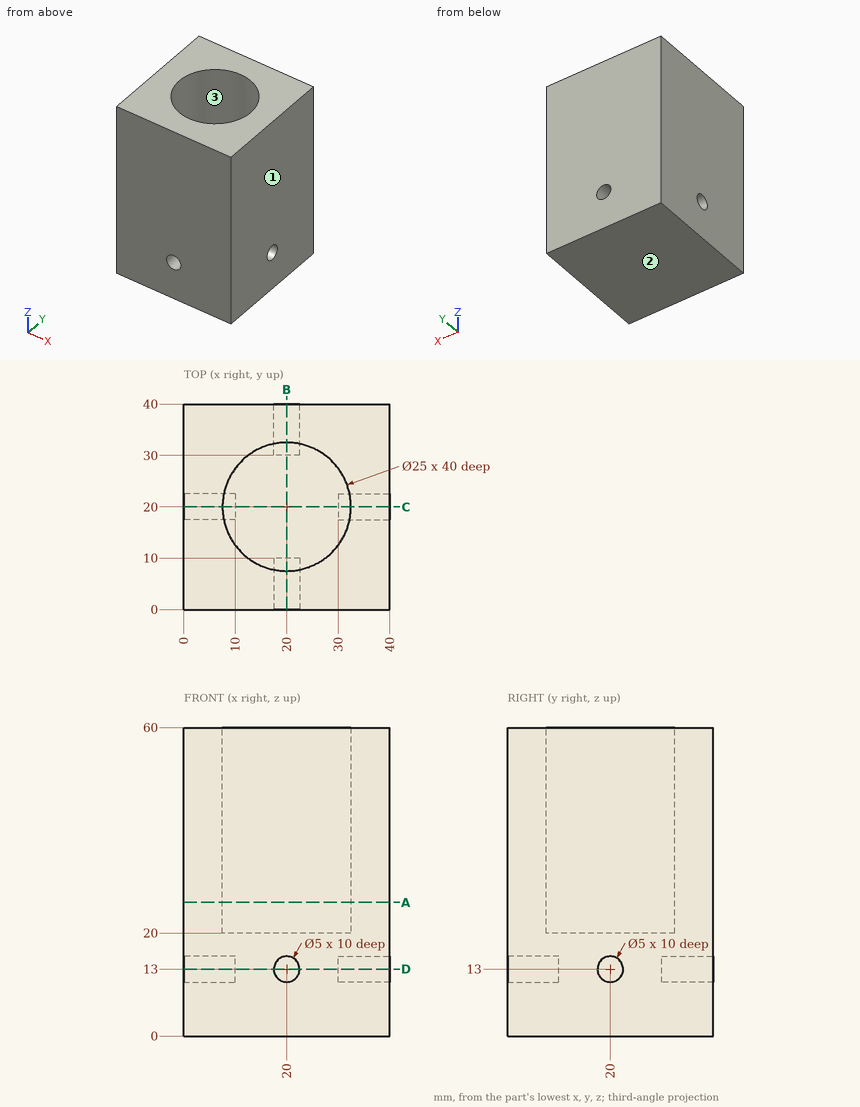
Answer from the drawing. Dimensions are ordinates in mm from the lowest x, y and z of the part. Give positions to 0.01 mm unless a question says otherwise; leave off trailing zeros. Order: outer loops, then holes, each group sorted by start corner. A loop starts at its lowest first (then second) coordinate and runs counter-clockwise, first axis right, second up. Notation, with made-up numbers: (-33, 63) -> (8, 63) arc R28 ccw to (8, 98) -> close; hole circle Ø10 at (21, 87.5). An arc over 180 degrees is marked (long way). One line per item, written item: value.
Item 1: Find section D-D, the plane z = 13. Give the vertices of the cut face in (x, y), plus the area to 3 significant figures.
Answer sheet:
outline: (0, 0) -> (17.5, 0) -> (17.5, 10) -> (22.5, 10) -> (22.5, 0) -> (40, 0) -> (40, 17.5) -> (30, 17.5) -> (30, 22.5) -> (40, 22.5) -> (40, 40) -> (22.5, 40) -> (22.5, 30) -> (17.5, 30) -> (17.5, 40) -> (0, 40) -> (0, 22.5) -> (10, 22.5) -> (10, 17.5) -> (0, 17.5) -> close
area: 1,400 mm²
Item 2: Find section A-A, the plane z = 26. Give the vertices of the cut face in (x, y).
Answer sheet:
outline: (0, 0) -> (40, 0) -> (40, 40) -> (0, 40) -> close; hole circle Ø25 at (20, 20)
Item 3: Flat-ended cylindrical pins translate along their axes: P1, Ø5, axis at x = 6, y = 8.5, coming from the -Z side; P2, Ø4, axis at y = 20, z = 13, coming from the +X side; P3, Ø12.5, axis at x = 19, y = 26, coming from the +Z side; P4, Ø1.5, axis at x = 19.5, z = 12, coming from the +Y side. Find the tip coordinate at first contact, or state that the pin passes through.
Answer sheet:
P1: z = 0
P2: x = 30
P3: z = 20
P4: y = 30
Item 4: Determine the mould class of the marked faces 1, 2 and 3 for opening direction X: released by +X, released by -X, zero draft, split by the parting line, or undercut.
Answer sheet:
face 1: released by +X
face 2: zero draft
face 3: undercut
Item 5: Straight lines are drawn through the part: probe 1 along Y at (x, z) = (12.5, 44.5); probe 2 along X at (y, z) = (35.75, 13); probe 3 along Y at (x, z) = (20, 31.5). For each, find the intervals that lie inside material, in ascending order.
Answer sheet:
probe 1: 0 to 10, 30 to 40
probe 2: 0 to 17.5, 22.5 to 40
probe 3: 0 to 7.5, 32.5 to 40
Item 6: Find section B-B, the plane x = 20. Give the vertices of the cut face in (y, z), plus the area to 3 significant figures.
Answer sheet:
outline: (0, 0) -> (40, 0) -> (40, 10.5) -> (30, 10.5) -> (30, 15.5) -> (40, 15.5) -> (40, 60) -> (32.5, 60) -> (32.5, 20) -> (7.5, 20) -> (7.5, 60) -> (0, 60) -> (0, 15.5) -> (10, 15.5) -> (10, 10.5) -> (0, 10.5) -> close
area: 1,300 mm²
